Check sheet for the modelled part. Datum: model origin and axes. Units: mm. A direction names the side the tool comes from. Coordinates: 2 decimals unless noted, no trailing zeros. Order: outer loops, then holes, each group sorted by start corner. A loop starts at its lowest first (then second) coordinate and runs counter-clockwise, first axis right, second up.
1. Cross-section at D-D (x = -4). Enter the section's corners in (y, z).
2. Gauge pin test, flat ends, axial feed: pin 1 Ø2 at (x, z) = (4, 1) entering from -Y; pin 2 Ø1 at (y, z) = (75.5, 0.5) entering from +X; pin 3 Ø1.6 at (y, z) = (60.5, 0.5) entering from -X; pin 4 Ø1.8 at (x, y) = (0, 67.91) entering from +Z. Record the tip position at first contact, or that the pin passes through.
3. Cross-section at B-B (z = 0.65). Enter the section's corners in (x, y), then the cut area to 3 significant figures.
4. Cross-section at A-A (x = 0). Enter the section's corners in (y, z).
5. Draft check along Y on faces 1 (the flat face through (0, 70, 0)), 2 (the flat face through (3, 72.956, 1)), 3 (the cylindrical face through (-0.51, 66.93, 1.97)). Enter one of: released by +Y, released by -Y, zero draft, split by the parting line, or undercut.
6. Set-up check for faces 4 (the flat face through (-3, 72.956, 1)), 5 (the flat face through (1.2, 70.3, 2)), 6 (the flat face through (-1.5, 60, 1)): record each of +Z, -Z, +X, -X, +Y, -Y from which the full face is reachable in a straight line by a thin tool's end or side.
7. Cross-section at C-C (y = 74.25). Enter the section's corners in (x, z).
8. Thickness scan on line 1 (Y direction, x = 0, z = 2.75); line 2 (Y direction, x = 0, z = 1); line 3 (X direction, y = 59.75, z = 1.2). Record the ranges inside material, lowest first.
Autodesk Inventor part; units mm, degrees
ref_plane "YZ Plane" through (0, 0, 0) normal (1, 0, 0) x (0, 1, 0)
ref_plane "XZ Plane" through (0, 0, 0) normal (0, 1, 0) x (-1, 0, 0)
ref_plane "XY Plane" through (0, 0, 0) normal (0, 0, 1) x (1, 0, 0)
sketch "Skizze1" plane through (0, 0, 0) normal (0, 0, 1) x (1, 0, 0)
  line L0 (2.8537, 62.8557) -> (-11.3867, 62.8557)
  line L1 (-8.4337, 63.8875) -> (2.8537, 63.8875)
  line L2 (2.8537, 63.8875) -> (2.8537, 62.8557)
  line L3 (5.1, 52.7557) -> (-5.1, 52.7557)
  line L4 (-5.1, 52.7557) -> (-5.1, 72.9557)
  line L5 (-5.1, 72.9557) -> (5.1, 72.9557)
  line L6 (5.1, 72.9557) -> (5.1, 52.7557)
  line L7 (5.1, 52.7557) -> (-5.1, 72.9557) construction
  line L8 (-5.1, 52.7557) -> (5.1, 72.9557) construction
  line L9 (5.1, 62.8557) -> (-5.1, 62.8557)
  point P0 (0, 0)
  point P1 (0, 62.8557)
extrude "Extrusion1" add sketch "Skizze1" along normal blind 2 contours L0 L4 L1 L2 | L2 L1 L4 L5 L6 L9
sketch "Skizze2" plane through (0, 0, 2) normal (0, 0, 1) x (1, 0, 0)
  line L0 (-5.1, 72.9557) -> (-5.1, 62.8557)
  line L1 (-5.1, 62.8557) -> (5.1, 62.8557)
  line L2 (5.1, 62.8557) -> (5.1, 72.9557)
  line L3 (5.1, 72.9557) -> (-5.1, 72.9557)
  circle A0 centre (0, 67.9057) radius 2.5
  circle A1 centre (0, 67.9057) radius 1.1
  point P0 (0, 0)
  dimension "d4" = 5
  dimension "d5" = 2.2
extrude "Extrusion2" add sketch "Skizze2" along normal blind 2 contours A0
sketch "Skizze3" plane through (0, 0, 2) normal (0, 0, 1) x (1, 0, 0)
  circle A0 centre (0, 67.9057) radius 1.1
  point P0 (0, 0)
extrude "Extrusion3" cut sketch "Skizze3" against normal blind 2
sketch "Skizze4" plane through (0, 0, 0) normal (0, 0, -1) x (-1, 0, 0)
  circle A0 centre (0, 67.9057) radius 1.1 construction
  line L0 (1.5, 77.9057) -> (-1.5, 77.9057)
  line L1 (-1.5, 77.9057) -> (-1.5, 57.9057)
  line L2 (-1.5, 57.9057) -> (1.5, 57.9057)
  line L3 (1.5, 57.9057) -> (1.5, 77.9057)
  line L4 (1.5, 77.9057) -> (-1.5, 57.9057) construction
  line L5 (-1.5, 77.9057) -> (1.5, 57.9057) construction
  point P0 (0, 0)
  dimension "d10" = 3
  dimension "d11" = 20
extrude "Extrusion4" add sketch "Skizze4" against normal blind 2
sketch "Skizze5" plane through (0, 0, 0) normal (0, 0, -1) x (-1, 0, 0)
  circle A0 centre (0, 67.9057) radius 1.1
  point P0 (0, 0)
extrude "Extrusion5" cut sketch "Skizze5" against normal blind 10
properties part number "amt_plate" material "Nylon 6/6"
Data:
1. outline: (62.86, 0) - (72.96, 0) - (72.96, 2) - (62.86, 2) - close
2. pin 1: stops at y = 62.86
2. pin 2: stops at x = 1.5
2. pin 3: stops at x = -1.5
2. pin 4: passes through
3. outline: (-5.1, 62.86) - (-1.5, 62.86) - (-1.5, 57.91) - (1.5, 57.91) - (1.5, 62.86) - (5.1, 62.86) - (5.1, 72.96) - (1.5, 72.96) - (1.5, 77.91) - (-1.5, 77.91) - (-1.5, 72.96) - (-5.1, 72.96) - close; hole circle Ø2.2 at (0, 67.91)
3. area: 129 mm2
4. outline: (57.91, 0) - (66.81, 0) - (66.81, 4) - (65.41, 4) - (65.41, 2) - (57.91, 2) - close; (69.01, 0) - (77.91, 0) - (77.91, 2) - (70.41, 2) - (70.41, 4) - (69.01, 4) - close
5. face 1: zero draft
5. face 2: released by +Y
5. face 3: undercut
6. face 4: +Z, -Z, -X, +Y
6. face 5: +Z
6. face 6: +Z, -Z, -X, -Y
7. outline: (-1.5, 0) - (1.5, 0) - (1.5, 2) - (-1.5, 2) - close
8. line 1: y = 65.41 to 66.81, 69.01 to 70.41
8. line 2: y = 57.91 to 66.81, 69.01 to 77.91
8. line 3: x = -1.5 to 1.5
